Work out the finished part from the listing and answer in its coordinate system (mm). A direction names the side the tool comes from. Round coordinates to 2 decimals unless told otherwise and drop trailing zeros. One line per item, written item: value. Start each with the question number.
Q1. Given pin 1 Ø6 at (y, z) = (81.5, 4) entering from +X; pin 2 Ø6 at (y, z) = (81.5, 10) entering from +X; pin 3 Ø1 at (x, z) = (92.5, 2) entering from +Y; pin 4 Ø2 at (x, z) = (42.5, 5.5) entering from +Y, each flat-ended and moving along its own axis, determine where each tip first touches the part or whether it passes through.
Q2. Consider probe 1 along Y at (x, z) = (24.5, 6.9); probe 2 along Y at (x, z) = (83, 9.2); probe 3 along Y at (x, z) = (83, 6.1). Determine where each line is inside the solid, lowest interval first.
Q3. A tool of negligible diameter and unlimited length cuts with its end or side. For faces 4 (the cylindrical face through (22.816, 73.72, 10.074)), 5 (the flat face through (23, 45, 10.5)), from which of +Z, -Z, +X, -X, +Y, -Y can it reach the whole face along a straight path? Write none if from no direction.
Q4. The mould has two halves that part along X. Classify faces 1 (the flat face through (62, 93.81, 6)), 2 (the flat face through (85.96, 73.13, 5.74)), 3 (the flat face through (65, 78, 4.5)): released by +X, released by -X, zero draft, split by the parting line, or undercut.
from build123d import *

# Parameters (mm, degrees)
BOSS_EXTRUDE1_DEPTH = 11.5
CUT_EXTRUDE1_DEPTH  = 10.5
CUT_EXTRUDE3_START  = 93.81
SKETCH10_R          = 1
CUT_EXTRUDE3_DEPTH  = 3
SKETCH11_R          = 5.15
CUT_EXTRUDE4_DEPTH  = 28.407206753
CUT_EXTRUDE6_START  = 11.5
CUT_EXTRUDE6_DEPTH  = 7
CUT_EXTRUDE10_START = 11.5
SKETCH17_R          = 1
CUT_EXTRUDE10_DEPTH = 7
CUT_EXTRUDE11_START = 11.5
CUT_EXTRUDE11_DEPTH = 1
FILLET1_R           = 5
FILLET2_R           = 5
SKETCH22_W          = 132.319501334
SKETCH22_H          = 14.071427362
CUT_EXTRUDE13_DEPTH = 143.060866263


with BuildPart() as part:
    # Sketch1 → Boss-Extrude1 (new body)
    with BuildSketch(Plane.XY):
        Polygon((0, 53.03), (49.407206753, 3.622793247), (56.652793247, 3.622793247), (106.06, 53.03), (65.28, 93.81), (61.03, 93.81), (61.03, 73.31), (45.03, 73.31), (45.03, 93.81), (40.78, 93.81), align=None)
    extrude(amount=BOSS_EXTRUDE1_DEPTH)

    # Sketch5 → Cut-Extrude1 (cut)
    with BuildSketch(Plane.XY.offset(11.5)):
        Polygon((26.07, 68.03), (32.07, 74.03), (73.99, 74.03), (79.99, 68.03), (79.99, 38.03), (73.99, 32.03), (32.07, 32.03), (26.07, 38.03), (26.07, 48.03), (11.07, 48.03), (11.07, 58.03), (26.07, 58.03), align=None)
    extrude(amount=-CUT_EXTRUDE1_DEPTH, mode=Mode.SUBTRACT)

    # Sketch10 → Cut-Extrude3 (cut)
    with BuildSketch(Plane(origin=(0, 0, 0), x_dir=(1, 0, 0), z_dir=(0, 1, 0)).offset(CUT_EXTRUDE3_START)):
        with Locations(Location((42.905, -5.75, 0), (0, 0, 270))):
            Circle(SKETCH10_R)
        with Locations(Location((63.155, -5.75, 0), (0, 0, 270))):
            Circle(SKETCH10_R)
    extrude(amount=-CUT_EXTRUDE3_DEPTH, mode=Mode.SUBTRACT)

    # Sketch11 → Cut-Extrude4 (cut)
    with BuildSketch(Plane.XZ.offset(-3.622793247)):
        with Locations(Location((53.03, 5.75, 0), (0, 0, 292.730860927))):
            Circle(SKETCH11_R)
    extrude(amount=-CUT_EXTRUDE4_DEPTH, mode=Mode.SUBTRACT)

    # Sketch13 → Cut-Extrude6 (cut)
    with BuildSketch(Plane.XY.offset(CUT_EXTRUDE6_START)):
        Polygon((73.99, 74.03), (61.03, 86.99), (61.03, 74.03), align=None)
        Polygon((32.07, 74.03), (45.03, 86.99), (45.03, 74.03), align=None)
    extrude(amount=-CUT_EXTRUDE6_DEPTH, mode=Mode.SUBTRACT)

    # Sketch17 → Cut-Extrude10 (cut)
    with BuildSketch(Plane.XY.offset(CUT_EXTRUDE10_START)):
        with Locations((24.5, 59.53)):
            Circle(SKETCH17_R)
        with Locations((24.5, 46.53)):
            Circle(SKETCH17_R)
        with Locations((83, 60.03)):
            Circle(SKETCH17_R)
        with Locations((83, 46.03)):
            Circle(SKETCH17_R)
    extrude(amount=-CUT_EXTRUDE10_DEPTH, mode=Mode.SUBTRACT)

    # Sketch19 → Cut-Extrude11 (cut)
    with BuildSketch(Plane.XY.offset(CUT_EXTRUDE11_START)):
        Polygon((13.96, 56.03), (13.96, 50.03), (32.07, 32.03), (73.99, 32.03), (95.1, 53.03), (73.99, 74.03), (32.07, 74.03), align=None)
    extrude(amount=-CUT_EXTRUDE11_DEPTH, mode=Mode.SUBTRACT)

    # Fillet1
    # the kernel refuses this fillet: 5 mm, written as the material it takes off along each edge
    with BuildSketch(Plane(origin=(47.813958483, -5.216041517, 11.5), x_dir=(0, 0, -1), z_dir=(0.7071067811865475, 0.7071067811865477, 0)), Plane(origin=(-8.838834765, 61.868834765, 11.5), x_dir=(0, 0, -1), z_dir=(0.7071067811865476, -0.7071067811865475, 0))) as fillet1_piece_1:
        with BuildLine():
            CenterArc((FILLET1_R, FILLET1_R), FILLET1_R, 180, 90)
            Line((0, FILLET1_R), (0, 0))
            Line((0, 0), (FILLET1_R, 0))
        make_face()
    extrude(amount=94.872341868, mode=Mode.SUBTRACT)
    with BuildSketch(Plane(origin=(49.618834765, 102.648834765, 11.5), x_dir=(0, 0, -1), z_dir=(-0.7071067811865472, -0.7071067811865479, 0)), Plane(origin=(114.898834765, 44.191165235, 11.5), x_dir=(0, 0, -1), z_dir=(-0.7071067811865476, 0.7071067811865476, 0))) as fillet1_piece_2:
        with BuildLine():
            CenterArc((FILLET1_R, FILLET1_R), FILLET1_R, 180, 90)
            Line((0, FILLET1_R), (0, 0))
            Line((0, 0), (FILLET1_R, 0))
        make_face()
    extrude(amount=82.671629074, mode=Mode.SUBTRACT)

    # Fillet2
    # the kernel refuses this fillet: 5 mm, written as the material it takes off along each edge
    with BuildSketch(Plane(origin=(49.618834765, 102.648834765, 0), x_dir=(0.7071067811865479, -0.7071067811865472, 0), z_dir=(-0.7071067811865472, -0.7071067811865479, 0)), Plane(origin=(114.898834765, 44.191165235, 0), x_dir=(-0.7071067811865476, -0.7071067811865476, 0), z_dir=(-0.7071067811865476, 0.7071067811865476, 0))) as fillet2_piece_1:
        with BuildLine():
            CenterArc((FILLET2_R, FILLET2_R), FILLET2_R, 180, 90)
            Line((0, FILLET2_R), (0, 0))
            Line((0, 0), (FILLET2_R, 0))
        make_face()
    extrude(amount=82.671629074, mode=Mode.SUBTRACT)
    with BuildSketch(Plane(origin=(-8.838834765, 61.868834765, 0), x_dir=(0, 0, 1), z_dir=(0.7071067811865476, -0.7071067811865475, 0))) as fillet2_piece_2:
        with BuildLine():
            CenterArc((FILLET2_R, -FILLET2_R), FILLET2_R, 90, 90)
            Line((0, -FILLET2_R), (0, 0))
            Line((0, 0), (FILLET2_R, 0))
        make_face()
    extrude(amount=94.872341868, mode=Mode.SUBTRACT)
    with BuildSketch(Plane(origin=(47.813958483, -5.216041517, 0), x_dir=(-0.7071067811865477, 0.7071067811865475, 0), z_dir=(0.7071067811865475, 0.7071067811865477, 0))) as fillet2_piece_3:
        with BuildLine():
            CenterArc((FILLET2_R, FILLET2_R), FILLET2_R, 180, 90)
            Line((0, FILLET2_R), (0, 0))
            Line((0, 0), (FILLET2_R, 0))
        make_face()
    extrude(amount=94.872341868, mode=Mode.SUBTRACT)

    # Sketch22 → Cut-Extrude13 (cut, through all)
    with BuildSketch(Plane.XY):
        Rectangle(SKETCH22_W, SKETCH22_H)
    extrude(amount=CUT_EXTRUDE13_DEPTH, mode=Mode.SUBTRACT)


solid = part.part
The answers:
1. pin 1: x = 80.51
1. pin 2: x = 79.6
1. pin 3: y = 65.87
1. pin 4: y = 93.81
2. probe 1: 28.55 to 45.53, 47.53 to 48.03, 58.03 to 58.53, 60.53 to 77.51
2. probe 2: 31.09 to 45.03, 47.03 to 59.03, 61.03 to 74.97
2. probe 3: 29.97 to 45.03, 47.03 to 59.03, 61.03 to 76.09
3. face 4: +Z, -X, +Y
3. face 5: +Z
4. face 1: zero draft
4. face 2: released by +X
4. face 3: undercut
